Autodesk Inventor part; units mm, degrees
ref_plane "Work Plane1" through (3, 0, 0) normal (1, 0, 0) x (0, 1, 0)
ref_plane "XZ Plane" through (0, 0, 0) normal (0, 1, 0) x (-1, 0, 0)
ref_plane "XY Plane" through (0, 0, 0) normal (0, 0, 1) x (1, 0, 0)
sketch "Sketch1" plane through (0, 0, 0) normal (0, 0, 1) x (1, 0, 0)
  line L0 (-25, 25) -> (25, 25)
  line L1 (25, 25) -> (25, -25)
  line L2 (25, -25) -> (-25, -25)
  line L3 (-25, -25) -> (-25, 25)
  point P0 (0, 0)
  point P1 (0, 25)
  dimension "d0" = 50
  dimension "d1" = 50
  dimension "d2" = 25
  dimension "d3" = 25
extrude "Extrusion1" add sketch "Sketch1" against normal blind 5
sketch "Sketch2" plane through (0, 0, 0) normal (0, 0, 1) x (1, 0, 0)
  circle A0 centre (0, 0) radius 3
  dimension "d6" = 6
extrude "Extrusion2" add sketch "Sketch2" along normal blind 7
ref_plane "Work Plane1" through (3, 0, 0) normal (1, 0, 0) x (0, 1, 0)
sketch "Sketch3" plane through (3, 0, 0) normal (1, 0, 0) x (0, 1, 0)
  point P0 (0, 0)
  point P1 (0, 4)
  dimension "d9" = 4
hole "Hole1" at (3, 0, 4) direction (-1, 0, 0) diameter 3 end through all
properties part number "Sampleholder1Thick"
Work out the finished part from the listing and answer in its coordinate system (mm). Coordinates: 2 decimals unless noted, no trailing zeros. Write each loop counter-clockwise with the first axis right and the second up, starting at its lowest first coordinate (ties: lowest second). Pieces come first, ordered by that corner, then holes. Notation, with made-up numbers: M 22.25,35.5 L 36.25,35.5 A32 ccw 36.25,72.5 Z; hole C -40,8 d11. An arc over 180 degrees is marked long. Use one line per item in the form item = value. Start each with the question number.
1. Each of these flat-tipped pins is pushed along its axis until it touches: P1, Ø3, axis at x = -0.5, z = 2, coming from the -Y side; P2, Ø5, axis at y = 0, z = 4, coming from the +X side. Where does it stop, or does it pass through?
2. The mould has two halves that part along Y. Classify faces 1 (the face through (0, 25, -2)), 2 (the face through (0, 0, 7)), 3 (the face through (-0.042, -1.265, 3.194)), 4 (the face through (-2.4, 1.8, 3.5)): released by +Y, released by -Y, zero draft, split by the parting line, or undercut.
3. The part is cut by section C-C (z = 6.25). Give the vertices of the cut face in (x, y).
4. The part is cut by section D-D (x = -18.5). Give the vertices of the cut face in (y, z).
5. Straight lines are drawn through the part: probe 1 along Z at (x, y) = (-1.5, 0); probe 2 along Y at (x, z) = (0.25, 4); probe 3 along Z at (x, y) = (-10.5, -13). For each, find the intervals that lie inside material, in ascending order. Write a range as from..to.
6. The part is cut by section A-A (x = 0). Give the vertices of the cut face in (y, z), plus the area to 3 significant figures.
7. The part is cut by section B-B (y = 0). Give the vertices of the cut face in (x, z), plus the area to 3 significant figures.
Evaluation:
q1.P1 = -3
q1.P2 = 3
q2.face_1 = released by +Y
q2.face_2 = zero draft
q2.face_3 = undercut
q2.face_4 = split by the parting line
q3.outline = C 0,0 d6
q4.outline = M -25,-5 L 25,-5 L 25,0 L -25,0 Z
q5.probe_1 = -5..2.5, 5.5..7
q5.probe_2 = -2.99..-1.5, 1.5..2.99
q5.probe_3 = -5..0
q6.outline = M -25,-5 L 25,-5 L 25,0 L 3,0 L 3,7 L -3,7 L -3,0 L -25,0 Z; hole C 0,4 d3
q6.area = 285 mm^2
q7.outline = M -25,-5 L 25,-5 L 25,0 L 3,0 L 3,2.5 L -3,2.5 L -3,0 L -25,0 Z; M -3,5.5 L 3,5.5 L 3,7 L -3,7 Z
q7.area = 274 mm^2
